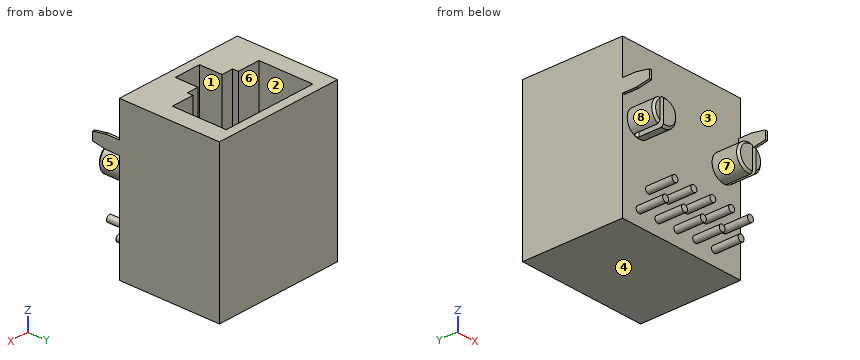
Autodesk Inventor part; units mm, degrees
ref_plane "YZ Plane" through (0, 0, 0) normal (1, 0, 0) x (0, 1, 0)
ref_plane "XZ Plane" through (0, 0, 0) normal (0, 1, 0) x (-1, 0, 0)
ref_plane "XY Plane" through (0, 0, 0) normal (0, 0, 1) x (1, 0, 0)
sketch "Sketch1" plane through (0, 0, 0) normal (0, 1, 0) x (-1, 0, 0)
  line L0 (7.95, 14.5) -> (-7.95, 14.5)
  line L1 (-7.95, 14.5) -> (-7.95, -4.3)
  line L2 (-7.95, -4.3) -> (7.95, -4.3)
  line L3 (7.95, -4.3) -> (7.95, 14.5)
  point P0 (0, 0)
  dimension "d0" = 18.8
  dimension "d1" = 15.9
  dimension "d2" = 7.95
  dimension "d5" = 14.5
extrude "Extrusion1" add sketch "Sketch1" along normal blind 12.25
sketch "Sketch2" plane through (-7.95, 0, 14.5) normal (0, 0, 1) x (1, 0, 0)
  line L0 (2.12, 11.155) -> (13.78, 11.155)
  line L1 (13.78, 11.155) -> (13.78, 4.555)
  line L2 (13.78, 4.555) -> (2.12, 4.555)
  line L3 (2.12, 4.555) -> (2.12, 11.155)
  line L4 (4.9, 4.555) -> (11, 4.555)
  line L5 (11, 4.555) -> (11, 3.865)
  line L6 (11, 3.865) -> (4.9, 3.865)
  line L7 (4.9, 3.865) -> (4.9, 4.555)
  line L8 (6.325, 3.865) -> (9.575, 3.865)
  line L9 (9.575, 3.865) -> (9.575, 1.095)
  line L10 (9.575, 1.095) -> (6.325, 1.095)
  line L11 (6.325, 1.095) -> (6.325, 3.865)
  line L12 (0, 12.25) -> (15.9, 12.25)
  point P0 (7.95, 0)
  dimension "d6" = 11.66
  dimension "d7" = 5.83
  dimension "d8" = 6.1
  dimension "d9" = 3.05
  dimension "d10" = 3.25
  dimension "d11" = 1.625
  dimension "d12" = 7.29
  dimension "d13" = 2.77
  dimension "d14" = 6.6
  dimension "d16" = 1.095
extrude "Extrusion2" cut sketch "Sketch2" against normal blind 12.32
sketch "Sketch3" plane through (7.95, 0, 14.5) normal (1, 0, 0) x (0, 0, -1)
  line L0 (4.3, 0) -> (5.9, 0)
  line L1 (5.9, 0) -> (5.9, -3.3)
  line L2 (5.9, -3.3) -> (4.3, -3.3)
  line L3 (4.3, -3.3) -> (4.3, 0)
  line L4 (0, 0) -> (0, 12.25)
  line L5 (4.3, -1.65) -> (4.5909, -3.3)
  line L6 (5.6091, -3.3) -> (5.9, -1.65)
  line L7 (0, 0) -> (18.8, 0)
  point P0 (14.5, 0)
  dimension "d19" = 3.3
  dimension "d20" = 1.6
  dimension "d21" = 4.3
  dimension "d22" = 10
  dimension "d23" = 10
  dimension "d24" = 1.65
  dimension "d25" = 0
extrude "Extrusion3" add sketch "Sketch3" against normal blind 0.3 contours L0 L1 L6 L2 L5 L3
mirror "Mirror1" about plane through (0, 0, 0) normal (1, 0, 0) of "Extrusion3"
sketch "Sketch4" plane through (0, 0, 0) normal (0, -1, 0) x (1, 0, 0)
  circle A0 centre (5.715, 6.35) radius 1.6
  line L0 (-7.95, 14.5) -> (7.95, 14.5)
  point P0 (0, 0)
  dimension "d28" = 3.2
  dimension "d29" = 8.15
  dimension "d30" = 5.715
extrude "Extrusion4" add sketch "Sketch4" along normal blind 3.25
chamfer "Chamfer1" distance 0.25 angle 45 1 edges at (4.115, -3.25, 6.35)
sketch "Sketch5" plane through (5.715, -3.25, 6.35) normal (0, -1, 0) x (1, 0, 0)
  line L0 (0.7635, 1.8366) -> (0.2859, 1.8366)
  line L1 (0.2859, 1.8366) -> (0.2859, -1.8337)
  line L2 (0.2859, -1.8337) -> (0.7635, -1.8337)
  line L3 (0.7635, -1.8337) -> (0.7635, 1.8366)
  point P0 (-5.715, -6.35)
extrude "Extrusion5" cut sketch "Sketch5" against normal blind 3.25
fillet "Fillet1" radius 0.25 1 edges at (6.0009, 0, 6.35)
fillet "Fillet2" radius 0.2 1 edges at (6.4785, 0, 6.35)
mirror "Mirror2" about plane through (0, 0, 0) normal (1, 0, 0) of "Extrusion4", "Chamfer1", "Extrusion5", "Fillet1", "Fillet2"
sketch "Sketch6" plane through (0, 0, 0) normal (0, -1, 0) x (1, 0, 0)
  line L0 (3.8973, 0) -> (-6.9227, 0) construction
  line L1 (4.2984, -2.54) -> (-6.5216, -2.54) construction
  circle A0 centre (0.635, 0) radius 0.4
  circle A1 centre (-0.635, -2.54) radius 0.4
  circle A2 centre (-3.175, -2.54) radius 0.4
  circle A3 centre (-5.715, -2.54) radius 0.4
  circle A4 centre (1.905, -2.54) radius 0.4
  circle A5 centre (-0.635, -2.54) radius 0.4
  circle A6 centre (-3.175, -2.54) radius 0.4
  circle A7 centre (4.445, -2.54) radius 0.4
  circle A8 centre (1.905, -2.54) radius 0.4
  circle A9 centre (-0.635, -2.54) radius 0.4
  circle A10 centre (-1.905, 0) radius 0.4
  circle A11 centre (-4.445, 0) radius 0.4
  circle A12 centre (3.175, 0) radius 0.4
  circle A13 centre (0.635, 0) radius 0.4
  circle A14 centre (-1.905, 0) radius 0.4
  circle A15 centre (5.715, 0) radius 0.4
  circle A16 centre (3.175, 0) radius 0.4
  circle A17 centre (0.635, 0) radius 0.4
  point P0 (0, 0)
  dimension "d40" = 2.54
  dimension "d41" = 0
  dimension "d45" = 0.8
  dimension "d46" = 0.8
  dimension "d49" = 2.54
  dimension "d52" = 2.54
  dimension "d57" = 2.54
  dimension "d60" = 2.54
  dimension "d63" = 0.635
  dimension "d64" = 0.635
extrude "Extrusion6" add sketch "Sketch6" along normal blind 3.25
properties part number "RJE051AA1310"
CAD build for the part. Positions are in the model's coordinates, mm. Face numbers are marked on the shaded views. A direction names the side the tool comes from. Give positions to 0.01 mm unless a question says otherwise; leave off trailing zeros. Loops run counter-clockwise (first coordinate to the right, second up) from the corner with the lowest first, then second, coordinate; pieces in that order, holes last. Notation, with made-up numbers: M 81.25,5 L 97.25,5 A17 cw 97.25,19 Z; hole C 60,40.5 d5. An arc over 180 degrees is marked long. Answer in a Markdown table with one row per item. Add a question column.
Item 1: Mould opens along Y. For the marked faces 1, 2, 3 and 4 say: +Y half, -Y half, draft (parallel to the pull), parting line (faces both ways), or undercut.
Item 2: Band-saw the part on A-A on z = 0. Give the cut face in (x, y) (3 decimals).
Item 3: Probe probe 1 along Y at (x, z) = (-2.25, 6.75) (3 decimals); probe 2 along Z at (x, y) = (5.75, -0.25); probe 3 along X at (y, z) = (7.5, 3.5). List the from-to ranges inside material, lowest first.
Item 4: Drop flat-ended pins along their axis: P1, Ø1.5, axis at x = 0.5, y = -1.5, coming from the +Z side; P2, Ø1.8, axis at x = 5, z = 6, coming from the -Y side. Give the stop position or say it passes through.
Item 5: Tool access for the marked faces 5, 6, 7 and 8: list every direction of +Z, -Z, +X, -X, +Y, -Y with a clear straight run to the whole face (end or side of a thin tool).
Item 6: Band-saw the part on B-B on y = 7.25. Give the cut face in (x, z).
Reply:
| question | item | result |
|---|---|---|
| 1 | face 1 | undercut |
| 1 | face 2 | undercut |
| 1 | face 3 | -Y half |
| 1 | face 4 | draft |
| 2 | outline | M -7.95,0 L -4.845,0 L -4.845,-3.25 L -4.045,-3.25 L -4.045,0 L -2.305,0 L -2.305,-3.25 L -1.505,-3.25 L -1.505,0 L 0.235,0 L 0.235,-3.25 L 1.035,-3.25 L 1.035,0 L 2.775,0 L 2.775,-3.25 L 3.575,-3.25 L 3.575,0 L 5.315,0 L 5.315,-3.25 L 6.115,-3.25 L 6.115,0 L 7.95,0 L 7.95,12.25 L -7.95,12.25 Z |
| 3 | probe 1 | y = 0 to 3.865, 11.155 to 12.25 |
| 3 | probe 2 | z = -0.4 to 0.4, 4.75 to 7.95 |
| 3 | probe 3 | x = -7.95 to -5.83, 5.83 to 7.95 |
| 4 | P1 | stops at z = 0.4 |
| 4 | P2 | stops at y = -3.25 |
| 5 | face 5 | +X, -Y |
| 5 | face 6 | +Z |
| 5 | face 7 | -Y |
| 5 | face 8 | -X, -Y |
| 6 | outline | M -7.95,-4.3 L 7.95,-4.3 L 7.95,14.5 L 5.83,14.5 L 5.83,2.18 L -5.83,2.18 L -5.83,14.5 L -7.95,14.5 Z |
